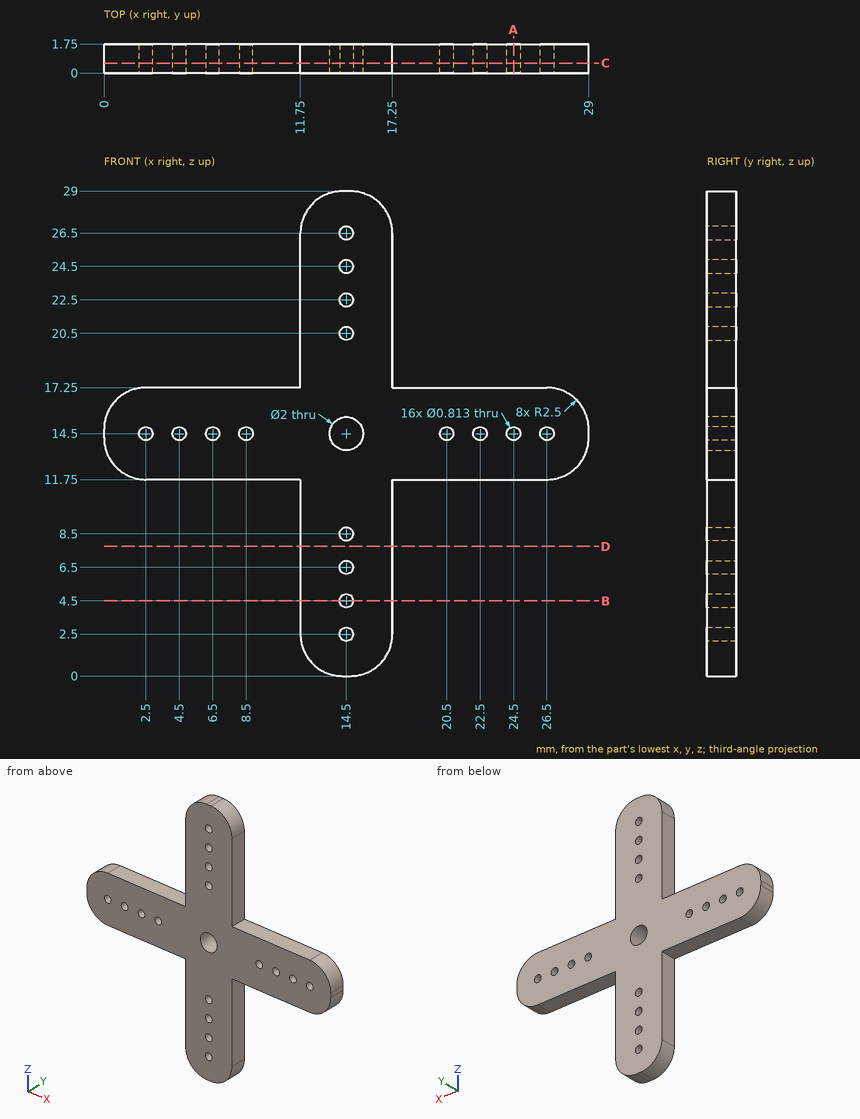
Check sheet for the drawn part. Datum: minimum x, y, z corner. Units: mm. Round coordinates to 2 decimals unless told otherwise and drop trailing zeros. Order: outer loops, then holes, each group sorted by start corner. A loop starts at its lowest first (then second) coordinate and runs counter-clockwise, first axis right, second up.
1) Section check B-B (z = 4.5). Record the boundary of the cut face in (x, y).
2) Go/stop test with flat-tipped pins: pin 1 Ø0.9 at (x, y) = (8, 1) entering from -Z; pin 2 Ø0.5 at (y, z) = (1, 21) entering from -X; pin 3 Ø0.5 at (y, z) = (0.5, 7) entering from +X. Record where each tip stops, or that it passes through.
3) Section check D-D (z = 7.75). Record the boundary of the cut face in (x, y).
4) Section check C-C (y = 0.6). Give the number of separate pieces and of enclosed holes in the cut face, and give its area (3 significant figures).
5) Section check A-A (x = 24.5). Record the boundary of the cut face in (y, z).
6) Scan line: line 1 (X direction, y = 0.4, z = 2.5). Record every from-to range of solid material in increasing order.
Result:
1. outline: (11.75, 0) - (14.09, 0) - (14.09, 1.75) - (11.75, 1.75) - close; (14.91, 0) - (17.25, 0) - (17.25, 1.75) - (14.91, 1.75) - close
2. pin 1: stops at z = 11.75
2. pin 2: stops at x = 11.75
2. pin 3: stops at x = 17.25
3. outline: (11.75, 0) - (17.25, 0) - (17.25, 1.75) - (11.75, 1.75) - close
4. separate pieces: 1
4. enclosed holes: 17
4. area: 267 mm2
5. outline: (0, 11.75) - (1.75, 11.75) - (1.75, 14.09) - (0, 14.09) - close; (0, 14.91) - (1.75, 14.91) - (1.75, 17.25) - (0, 17.25) - close
6. line 1: x = 11.75 to 14.09, 14.91 to 17.25
